from build123d import *

# Parameters (mm, degrees)
F1_DEPTH = 6.35


with BuildPart() as f1:
    # F0 (on Front) → F1 (new body, symmetric)
    with BuildSketch(Plane.XZ):
        Polygon((12.08981, 28.207475), (15.632335, 31.75), (-15.632335, 31.75), (-12.08981, 28.207475), (-19.45362, 20.843665), (-22.225, 23.615045), (-22.225, -23.615045), (-19.45362, -20.843665), (-12.08981, -28.207475), (-15.632335, -31.75), (15.632335, -31.75), (12.08981, -28.207475), (19.45362, -20.843665), (22.225, -23.615045), (22.225, 23.615045), (19.45362, 20.843665), align=None)
        Polygon((-22.225, 31.75), (-15.632335, 31.75), (-33.642425, 49.76009), (-41.006235, 42.39628), (-22.225, 23.615045), align=None)
        Polygon((41.006235, -42.39628), (22.225, -23.615045), (22.225, -31.75), (15.632335, -31.75), (33.642425, -49.76009), align=None)
        Polygon((-22.225, -31.75), (-22.225, -23.615045), (-41.006235, -42.39628), (-33.642425, -49.76009), (-15.632335, -31.75), align=None)
        Polygon((15.632335, 31.75), (22.225, 31.75), (22.225, 23.615045), (41.006235, 42.39628), (33.642425, 49.76009), align=None)
        Polygon((22.225, -31.75), (22.225, -23.615045), (19.45362, -20.843665), (12.08981, -28.207475), (15.632335, -31.75), align=None)
        Polygon((-19.45362, -20.843665), (-22.225, -23.615045), (-22.225, -31.75), (-15.632335, -31.75), (-12.08981, -28.207475), align=None)
        Polygon((-12.08981, 28.207475), (-15.632335, 31.75), (-22.225, 31.75), (-22.225, 23.615045), (-19.45362, 20.843665), align=None)
        Polygon((22.225, 23.615045), (22.225, 31.75), (15.632335, 31.75), (12.08981, 28.207475), (19.45362, 20.843665), align=None)
    extrude(amount=F1_DEPTH, both=True)


solid = f1.part
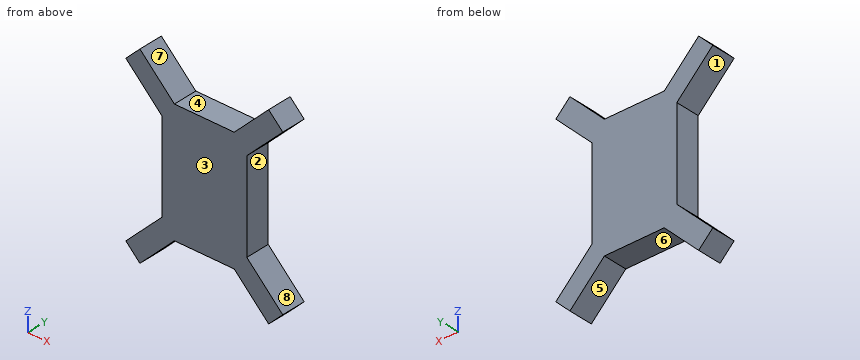
Could you check a few things on this model? Use its own coordinates, in mm. Face numbers are marked on the shaded views. A direction names the side the tool comes from. Give positions to 0.01 mm unless a question says otherwise; leave off trailing zeros. Order: outer loops, then holes, each group sorted by start corner. A loop starts at its lowest first (then second) coordinate and runs counter-clockwise, first axis right, second up. Notation, with made-up numbers: (41, 22) - (87, 22) arc R23 ccw to (87, 38) - close; hole circle Ø8 at (29.25, -3). An arc over 180 degrees is marked (long way). One line per item, written item: value. Start each with the question number.
1. Thinking about a two-plate mould opening in Z: for the marked faces 6, 7 and 8, which applies, +Z half, -Z half, draft (parallel to the pull), parting line (faces both ways), or undercut?
2. Imagine slicing it at B-B on x = -35. List the corners of the cut face in (y, z) for me, plus the area to 3 significant figures.
3. Imagine slicing it at A-A on z = 39.5. List the corners of the cut face in (x, y) for me, plus the area to 3 significant figures.
4. For the marked faces 1, 2, 3, 4 and 5, which set-ups out of +Z, -Z, +X, -X, +Y, -Y let a thin tool reach every point of the face, with its end or its side?
5. If I drill on probe 1 along X at (y, z) = (4.25, 1.5) (3 decimals); probe 2 along Z at (x, y) = (35, -0.25); probe 3 along X at (y, z) = (-3, -44.5), over which ranges is the centre line in solid material (lowest first)?
6. For P1, Ø6.5, axis at x = -2.5, y = 2.5, coming from the -Z side; P2, Ø4, axis at y = -3, z = 1, coming from the -X side (3 decimals); P3, Ø4, axis at x = 10, y = 2.5, coming from the +Z side, each with a flat end and sliding along its axis, tell me the tip position at first contact or that it passes through.
7. Imagine slicing it at D-D on z = -12. List the corners of the cut face in (x, y) for me (3 decimals), plus the area to 3 significant figures.
8. Imagine slicing it at C-C on y = -4. List the corners of the cut face in (x, z) for me (3 decimals), plus the area to 3 significant figures.
Values:
1. face 6: -Z half
1. face 7: +Z half
1. face 8: undercut
2. outline: (-6.35, -48.4) - (6.35, -48.4) - (6.35, -36.39) - (-6.35, -36.39) - close; (-6.35, 36.39) - (6.35, 36.39) - (6.35, 48.4) - (-6.35, 48.4) - close
2. area: 305 mm²
3. outline: (-38.11, -6.35) - (-23.38, -6.35) - (-23.38, 6.35) - (-38.11, 6.35) - close; (23.38, -6.35) - (38.11, -6.35) - (38.11, 6.35) - (23.38, 6.35) - close
3. area: 374 mm²
4. face 1: -X, +Y, -Y
4. face 2: +X, +Y, -Y
4. face 3: +Z, -Z, +X, -X, -Y
4. face 4: +Z, +Y, -Y
4. face 5: -Z, +Y, -Y
5. probe 1: -22.225 to 22.225
5. probe 2: -48.4 to -36.39, 36.39 to 48.4
5. probe 3: -38.9 to -28.38, 28.38 to 38.9
6. P1: z = -31.75
6. P2: x = -22.225
6. P3: z = 31.75
7. outline: (-22.225, -6.35) - (22.225, -6.35) - (22.225, 6.35) - (-22.225, 6.35) - close
7. area: 565 mm²
8. outline: (-41.006, -42.396) - (-33.642, -49.76) - (-15.632, -31.75) - (15.632, -31.75) - (33.642, -49.76) - (41.006, -42.396) - (22.225, -23.615) - (22.225, 23.615) - (41.006, 42.396) - (33.642, 49.76) - (15.632, 31.75) - (-15.632, 31.75) - (-33.642, 49.76) - (-41.006, 42.396) - (-22.225, 23.615) - (-22.225, -23.615) - close
8. area: 3,800 mm²
